Autodesk Inventor part; units mm, degrees
ref_plane "YZ Plane" through (0, 0, 0) normal (1, 0, 0) x (0, 1, 0)
ref_plane "XZ Plane" through (0, 0, 0) normal (0, 1, 0) x (-1, 0, 0)
ref_plane "XY Plane" through (0, 0, 0) normal (0, 0, 1) x (1, 0, 0)
sketch "Sketch1" plane through (0, 0, 0) normal (0, 1, 0) x (-1, 0, 0)
  line L0 (19, 0) -> (0, 0)
  line L1 (0, 0) -> (0, -38)
  line L2 (0, -38) -> (19, -38)
  line L3 (19, -38) -> (19, 0)
  line L4 (21, 2) -> (-2, 2)
  line L5 (-2, 2) -> (-2, -40)
  line L6 (-2, -40) -> (21, -40)
  line L7 (21, -40) -> (21, 2)
  dimension "d0" = 19
  dimension "d1" = 38
  dimension "d2" = 90
  dimension "d3" = 90
  dimension "d9" = 42
  dimension "d10" = 2
  dimension "d11" = 2
  dimension "d12" = 2
  dimension "d30" = 22
extrude "Extrusion1" add sketch "Sketch1" against normal blind 2 contours L3 L2 L1 L0 | L7 L6 L5 L4
sketch "Sketch2" plane through (0, 0, 0) normal (0, 1, 0) x (1, 0, 0)
  line L0 (0, 0) -> (0, 38)
  line L1 (0, 38) -> (-19, 38)
  line L2 (-19, 38) -> (-19, 0)
  line L3 (-19, 0) -> (0, 0)
  line L4 (-21, 40) -> (-21, -2)
  line L5 (2, 40) -> (-21, 40)
  line L6 (2, -2) -> (-21, -2)
  line L7 (-21, -2) -> (2, -2)
  line L8 (2, -2) -> (2, 40)
  line L9 (2, 40) -> (-21, 40)
  point P0 (2, 40)
  dimension "d15" = 2
  dimension "d16" = 2
  dimension "d17" = 90
extrude "Extrusion2" add sketch "Sketch2" along normal blind 15
sketch "Sketch3" plane through (0, -2, 0) normal (0, -1, 0) x (1, 0, 0)
  circle A0 centre (-9, -19) radius 22.5 construction
  circle A1 centre (-24.9099, -3.0901) radius 2.5
  circle A2 centre (6.9099, -34.9099) radius 2.5
  line L0 (-24.9099, -3.0901) -> (6.9099, -34.9099) construction
  circle A3 centre (6.9099, -3.0901) radius 2.5
  line L1 (-24.9099, -34.9099) -> (6.9099, -3.0901) construction
  circle A4 centre (-24.9099, -34.9099) radius 2.5
  line L2 (-9, 3.5) -> (-9, -41.5) construction
  line L3 (2, -40) -> (2, 2)
  line L4 (-21, -40) -> (2, -40)
  line L5 (-21, 2) -> (-30, 2)
  line L6 (-30, 2) -> (-30, -40)
  line L7 (-30, -40) -> (-21, -40)
  line L8 (2, -40) -> (11, -40)
  line L9 (11, -40) -> (11, 2)
  line L10 (11, 2) -> (2, 2)
  line L11 (-21, 2) -> (-21, -40)
  point P0 (0, 0)
  point P1 (-9, -19)
  point P2 (-9, -19)
  dimension "d20" = 45
  dimension "d21" = 5
  dimension "d22" = 5
  dimension "d23" = 45
  dimension "d24" = 5
  dimension "d25" = 5
  dimension "d26" = 45
  dimension "d27" = 90
  dimension "d28" = 45
  dimension "d29" = 11
  dimension "d31" = 21
  dimension "d32" = 0
  dimension "d33" = 9
  dimension "d34" = 42
  dimension "d35" = 9
extrude "Extrusion3" add sketch "Sketch3" against normal blind 5
fillet "Fillet1" radius 2 4 edges at (11, 0.5, 2) (11, 0.5, -40) (-30, 0.5, -40) (-30, 0.5, 2)
properties part number "Teenscy Holder"
Check sheet for the modelled part. Datum: model origin and axes. Units: mm. A direction names the side the tool comes from. Give positions to 0.01 mm unless a question says otherwise; leave off trailing zeros. Write each loop counter-clockwise with the first axis right and the second up, starting at its lowest first coordinate (ties: lowest second). Pieces come first, ordered by that corner, then holes.
Item 1: Cross-section at B-B (z = -2). Enter the section's corners in (x, y).
Item 2: Scan lines: L1, parallel to X at y = 7, z = -7.5; L2, parallel to Z at x = -13.5, y = 5.25; L3, parallel to X at y = 0.5, z = -18. Record each from-to range of solid material in increasing order.
Item 3: Cross-section at C-C (x = -23). Enter the section's corners in (y, z), and give its area (3 significant figures).
Item 4: Gauge pin test, flat ends, axial feed: pin 1 (4 mm diameter, centred on x = -6, z = -35, fed in from +Y); pin 2 (9.5 mm diameter, centred on y = 9, z = -29.5, fed in from -X); pin 3 (6.5 mm diameter, centred on x = -24.91, z = -34.91, fed in from +Y). Record the tip position at first contact, or that the pin passes through.
Item 5: Access from +Z, -Z, +X, -X, +Y, -Y to the whole of each face (thin tool, end or side, straight path). Record for faces 4 (the face through (-21, 9, -19)), 5 (the face through (-9, 0, -19)), 6 (the face through (6, 3, -19)).
Item 6: Cross-section at A-A (y = 12.75). Enter the section's corners in (x, z), and give its area (3 significant figures).
Item 7: Draft check along X on faces 1 (the face through (-29.4, 0.54, -39.43)), 2 (the face through (-20, 15, -21)), 3 (the face through (0, 7, -19)). Enter one of: released by +X, released by -X, zero draft, split by the parting line, or undercut.
Item 8: Cross-section at D-D (x = -17). Enter the section's corners in (y, z), and give its area (3 significant figures).
Report:
1. outline: (-30, -2) - (-27.16, -2) - (-27.16, 3) - (-30, 3) - close; (-22.66, -2) - (4.66, -2) - (4.66, 3) - (2, 3) - (2, 15) - (0, 15) - (0, 0) - (-19, 0) - (-19, 15) - (-21, 15) - (-21, 3) - (-22.66, 3) - close; (9.16, -2) - (11, -2) - (11, 3) - (9.16, 3) - close
2. L1: x = -21 to -19, 0 to 2
2. L2: z = -40 to -38, 0 to 2
2. L3: x = -30 to -19, 0 to 11
3. outline: (-2, -40) - (3, -40) - (3, -36.52) - (-2, -36.52) - close; (-2, -33.3) - (3, -33.3) - (3, -4.7) - (-2, -4.7) - close; (-2, -1.48) - (3, -1.48) - (3, 2) - (-2, 2) - close
3. area: 178 mm2
4. pin 1: stops at y = 0
4. pin 2: stops at x = -21
4. pin 3: stops at y = 3
5. face 4: +Z, -Z, -X, +Y
5. face 5: +Y
5. face 6: +Z, -Z, +X, +Y
6. outline: (-21, -40) - (2, -40) - (2, 2) - (-21, 2) - close; hole (-19, -38) - (0, -38) - (0, 0) - (-19, 0) - close
6. area: 244 mm2
7. face 1: released by -X
7. face 2: zero draft
7. face 3: undercut
8. outline: (-2, -40) - (15, -40) - (15, -38) - (0, -38) - (0, 0) - (15, 0) - (15, 2) - (-2, 2) - close
8. area: 144 mm2
